```python
from build123d import *

# Parameters (mm, degrees)
SKIZZE1_W                       = 90
SKIZZE1_H                       = 31
AUFSATZ_LINEAR_AUSTRAGEN1_DEPTH = 4
SKIZZE4_R                       = 8.85
SKIZZE4_R_2                     = 2.55
AUFSATZ_LINEAR_AUSTRAGEN3_DEPTH = 4
LINEARES_MUSTER1_COUNT          = 2
LINEARES_MUSTER1_PITCH          = 58
VERRUNDUNG2_R                   = 10
VERRUNDUNG3_R                   = 2
SKIZZE6_R                       = 1.55
SCHNITT_LINEAR_AUSTRAGEN1_DEPTH = 4
VERRUNDUNG4_R                   = 1


with BuildPart() as part:
    # Skizze1 → Aufsatz-Linear austragen1 (new body)
    with BuildSketch(Plane.XY):
        with Locations((-4.068471812, 5.991025438)):
            Rectangle(SKIZZE1_W, SKIZZE1_H)
    extrude(amount=AUFSATZ_LINEAR_AUSTRAGEN1_DEPTH)

    # Skizze4 → Aufsatz-Linear austragen3 (add)
    with BuildSketch(Plane(origin=(26.931528188, 0, 0), x_dir=(0, 0, -1), z_dir=(1, 0, 0))):
        with Locations((-2, -18.01992615)):
            Circle(SKIZZE4_R)
        with Locations((-2, -18.01992615)):
            Circle(SKIZZE4_R_2, mode=Mode.SUBTRACT)
    aufsatz_linear_austragen3 = extrude(amount=-AUFSATZ_LINEAR_AUSTRAGEN3_DEPTH)

    # Lineares Muster1: Aufsatz-Linear austragen3 ×2
    with Locations(*[(-i * LINEARES_MUSTER1_PITCH, 0, 0) for i in range(1, LINEARES_MUSTER1_COUNT)]):
        add(aufsatz_linear_austragen3)

    # Verrundung2
    verrundung2_edges = [part.edges().sort_by_distance(p)[0] for p in [
        (24.931528188, -9.39887633, 4),
        (-33.068471812, -9.39887633, 4),
    ]]
    fillet(verrundung2_edges, radius=VERRUNDUNG2_R)

    # Verrundung3
    verrundung3_edges = [part.edges().sort_by_distance(p)[0] for p in [
        (24.931528188, -9.39887633, 0),
        (-33.068471812, -9.39887633, 0),
    ]]
    fillet(verrundung3_edges, radius=VERRUNDUNG3_R)

    # Skizze6 → Schnitt-Linear austragen1 (cut)
    with BuildSketch(Plane.XY.offset(4)):
        with Locations((-26.568471812, 7.991025438)):
            Circle(SKIZZE6_R)
        with Locations((18.431528188, 7.991025438)):
            Circle(SKIZZE6_R)
    extrude(amount=-SCHNITT_LINEAR_AUSTRAGEN1_DEPTH, mode=Mode.SUBTRACT)

    # Verrundung4
    verrundung4_edges = [part.edges().sort_by_distance(p)[0] for p in [
        (40.931528188, -9.508974562, 2),
        (-49.068471812, -9.508974562, 2),
        (-49.068471812, 21.491025438, 2),
        (40.931528188, 21.491025438, 2),
    ]]
    fillet(verrundung4_edges, radius=VERRUNDUNG4_R)


solid = part.part
```
Geometry: final body of the model. Coordinates: model frame, mm. A direction names the side the tool comes from. Coordinates: 2 decimals unless noted, no trailing zeros. Order: outer loops, then holes, each group sorted by start corner. A loop starts at its lowest first (then second) coordinate and runs counter-clockwise, first axis right, second up. Notation, with made-up numbers: (20.5, 45) - (59.5, 45) arc R4 cw to (59.5, 52) - close; hole circle Ø1 at (-20, 85). An arc over 180 degrees is marked (long way). Write each question's results on one line, items separated by ' | '.
1) Pin query (flat end, axial travel): pin 1 (1 mm diameter, centred on x = -31.5, z = 8.5, fed in from +Y); pin 2 (3 mm diameter, centred on x = 33.5, z = 1, fed in from -Y); pin 3 (5.5 mm diameter, centred on y = -15.5, z = -2, fed in from +X). Return the tip coordinate at first contact, or that it passes through.
Results list:
pin 1: y = -11.51 | pin 2: y = -9.51 | pin 3: x = 26.93
2) Section B-B, the plane z = -5.25. Return loops of the section in (x, y), plus the area to 3 significant figures.
Results list:
outline: (-35.07, -23.1) - (-31.07, -23.1) - (-31.07, -12.94) - (-35.07, -12.94) - close; (22.93, -23.1) - (26.93, -23.1) - (26.93, -12.94) - (22.93, -12.94) - close | area: 81.2 mm^2
3) Line query: line 1 (X direction, y = -15, z = 5); line 2 (Y direction, x = -31.9, z = 2); line 3 (Z direction, x = 17, y = 12.5). Output: solid intervals per line, ascending. Write a range as from..to.
Results list:
line 1: -35.07..-31.07, 22.93..26.93 | line 2: -26.87..-20.57, -15.47..21.49 | line 3: 0..4
4) Section A-A, the plane z = 2.5. Return loops of the section in (x, y), plus the area to 3 significant figures.
Results list:
outline: (-49.07, -8.51) arc R1 ccw to (-48.07, -9.51) - (-35.07, -9.51) - (-35.07, -15.52) - (-31.07, -15.52) - (-31.07, -9.51) - (22.93, -9.51) - (22.93, -15.52) - (26.93, -15.52) - (26.93, -9.51) - (39.93, -9.51) arc R1 ccw to (40.93, -8.51) - (40.93, 20.49) arc R1 ccw to (39.93, 21.49) - (-48.07, 21.49) arc R1 ccw to (-49.07, 20.49) - close; (-35.07, -26.86) - (-31.07, -26.86) - (-31.07, -20.52) - (-35.07, -20.52) - close; (22.93, -26.86) - (26.93, -26.86) - (26.93, -20.52) - (22.93, -20.52) - close; hole circle Ø3.1 at (-26.57, 7.99); hole circle Ø3.1 at (18.43, 7.99) | area: 2,870 mm^2
5) Section C-C, the plane y = -23. Return loops of the section in (x, z), plus the area to 3 significant figures.
Results list:
outline: (-35.07, -5.32) - (-31.07, -5.32) - (-31.07, 9.32) - (-35.07, 9.32) - close; (22.93, -5.32) - (26.93, -5.32) - (26.93, 9.32) - (22.93, 9.32) - close | area: 117 mm^2
6) Section D-D, the plane x = 25. Return loops of the section in (y, z).
Results list:
outline: (-11.19, 7.63) arc R8.85 ccw (long way) to (-9.79, -1.26) arc R2 cw to (-7.93, 0) - (21.49, 0) - (21.49, 4) - (-3.48, 4) arc R10 cw to start; hole circle Ø5.1 at (-18.02, 2)
7) Set-up query: faces 5 (the cylindrical face through (24.96, -7.8, 4.98)), 6 (the flat face through (-42, -9.509, 2)), 7 (the flat face through (-5, 6, 4)), 8 (the flat face through (-4, -9.509, 2)), 9 (the flat face through (33, -9.509, 2)). Return all of +Z, -Z, +X, -X, +Y, -Y with unobstructed straight access to the full face (end or side cutting, diameter ignored); none if empty.
Results list:
face 5: +Z, +X, -X, +Y | face 6: +Z, -Z, -X, -Y | face 7: +Z, +Y | face 8: +Z, -Z, -Y | face 9: +Z, -Z, +X, -Y
8) Pull-direction query (Z, two-part tool) for faces 1 (the cylindrical face through (19.863, 7.397, 2.028)), 2 (the cylindrical face through (-33.04, -9.072, -0.355)), 3 (the cylindrical face through (-33.04, -17.908, 4.548)), 4 (the cylindrical face through (25, -26.8, 0.9)); classes: pulls with the +Z half, pulls with the -Z half, needs draft (parallel to the pull), parting line crosses it, or undercut.
Results list:
face 1: needs draft | face 2: pulls with the -Z half | face 3: undercut | face 4: parting line crosses it
